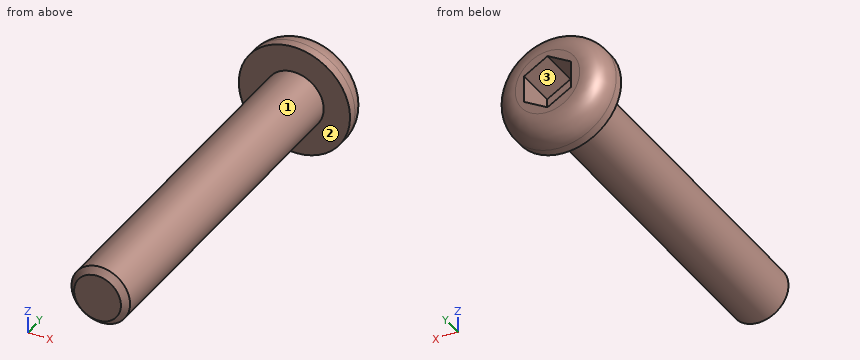
from build123d import *

# Parameters (mm, degrees)
CORTAR_EXTRUIR1_DEPTH = 3.5
CHAFL_N1_SIZE         = 0.5
REDONDEO1_R           = 2


with BuildPart() as part:
    # Croquis1 → Revolución1 (revolve)
    with BuildSketch(Plane.XY):
        Polygon((0, 0), (4.75, 0), (4.75, -2.75), (2.5, -2.75), (2.5, -32.75), (0, -32.75), align=None)
    revolve(axis=Axis((0, 0, 0), (0, -1, 0)))

    # Croquis2 → Cortar-Extruir1 (cut)
    with BuildSketch(Plane(origin=(0, 0, 0), x_dir=(1, 0, 0), z_dir=(0, 1, 0))):
        Polygon((2, 1.154700538), (0, 2.309401077), (-2, 1.154700538), (-2, -1.154700538), (0, -2.309401077), (2, -1.154700538), align=None)
    extrude(amount=-CORTAR_EXTRUIR1_DEPTH, mode=Mode.SUBTRACT)

    # Chaflán1
    chafl_n1_edges = [part.edges().sort_by_distance(p)[0] for p in [
        (-2.5, -32.75, 0),
    ]]
    chamfer(chafl_n1_edges, length=CHAFL_N1_SIZE)

    # Redondeo1
    redondeo1_edges = [part.edges().sort_by_distance(p)[0] for p in [
        (-4.75, 0, 0),
    ]]
    fillet(redondeo1_edges, radius=REDONDEO1_R)


solid = part.part
For this review, take the finished solid that the model builds, in its own axes (mm). Face numbers are marked on the shaded views. Round coordinates to 2 decimals unless told otherwise and drop trailing zeros. Order: outer loops, then holes, each group sorted by start corner. A loop starts at its lowest first (then second) coordinate and runs counter-clockwise, first axis right, second up. Notation, with made-up numbers: M 68.5,70.5 L 103.5,70.5 A15 cw 103.5,74.5 Z; hole C -2,31 d2. An arc over 180 degrees is marked long. Write each question's results on one line, items separated by ' | '. Start each with the question number.
1. Clearance check with flat-ended pins moving along their axes: pin 1 Ø3 at (x, y) = (0, -15.5) entering from -Z; pin 2 Ø1.2 at (x, z) = (-0.5, 0) entering from +Y; pin 3 Ø2 at (y, z) = (-8, 3) entering from +X. State where each tip first meets the part, or that it passes through.
2. Draft analysis for pull direction X (two halves, no side actions). For the marked faces 1, 2 and 3, state which applies: pulls with the +X half, pulls with the -X half, needs draft (parallel to the pull), parting line crosses it, or undercut.
3. To check wall thickness, follow L1, parallel to Y at x = -1.75, z = 0.5; L2, parallel to X at y = -19, z = 1.5. State the ranges of each line that lie inside material, in increasing order. Write a range as [from, to].
4. Add section A-A (z = 0). State the section outline as (x, y) points.
5. Add section B-B (y = -15.5). State the section outline as (x, z) points, then the cut area to 3 significant figures.
Output values:
1) pin 1: z = -2.5 | pin 2: y = -3.5 | pin 3: x = 1.5
2) face 1: parting line crosses it | face 2: needs draft | face 3: undercut
3) L1: [-32.75, -3.5] | L2: [-2, 2]
4) outline: M -4.75,-2.75 L -2.5,-2.75 L -2.5,-32.25 L -2,-32.75 L 2,-32.75 L 2.5,-32.25 L 2.5,-2.75 L 4.75,-2.75 L 4.75,-2 A2 ccw 2.75,0 L 2,0 L 2,-3.5 L -2,-3.5 L -2,0 L -2.75,0 A2 ccw -4.75,-2 Z
5) outline: C 0,0 d5 | area: 19.6 mm^2
